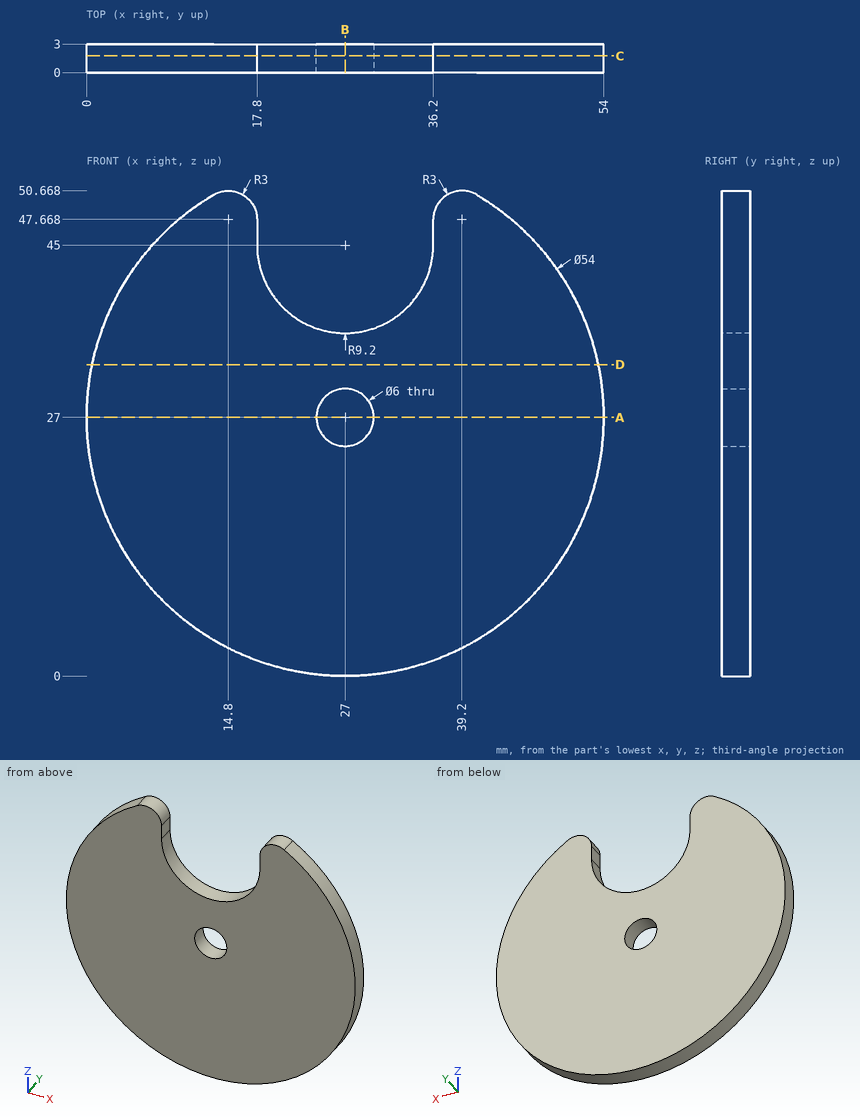
Job drawing, mm, ordinate dimensions from the low corner. One solid piece. Round coordinates to 2 decimals unless told otherwise and drop trailing zeros. Loops run counter-clockwise (first coordinate to the right, second up) from the corner with the lowest first, then second, coordinate; pieces in that order, holes last.
Item 1: Cut at A-A, the plane z = 27. Give the cut face in (x, y), then the cut area to 3 significant figures.
Item 2: Cut at D-D, the plane z = 32.5. Give the cut face in (x, y).
Item 3: Cut at B-B, the plane x = 27. Give the cut face in (y, z), then the cut area to 3 significant figures.
Item 4: Cut at C-C, the plane y = 1.75. Give the cut face in (x, z) (1 decimal), then the cut area to 3 significant figures.
Item 5: Drop a flat-ended pin along its axis: P1, Ø1.3, axis at y = 2, z = 46.5, coming from the -X side. Give the stop position or say it passes through.
Item 6: Drill centre lines: line 1 (Z direction, x = 27, y = 0.95); line 2 (Z direction, x = 29, y = 1.3) (1 decimal); line 3 (X direction, y = 0.55, z = 41.5). Where is each one in solid material? Low to high.
A:
1. outline: (0, 0) - (24, 0) - (24, 3) - (0, 3) - close; (30, 0) - (54, 0) - (54, 3) - (30, 3) - close
1. area: 144 mm2
2. outline: (0.57, 0) - (53.43, 0) - (53.43, 3) - (0.57, 3) - close
3. outline: (0, 0) - (3, 0) - (3, 24) - (0, 24) - close; (0, 30) - (3, 30) - (3, 35.8) - (0, 35.8) - close
3. area: 89.4 mm2
4. outline: (13.3, 50.3) arc R27 ccw (long way) to (40.7, 50.3) arc R3 ccw to (36.2, 47.7) - (36.2, 45) arc R9.2 cw to (17.8, 45) - (17.8, 47.7) arc R3 ccw to start; hole circle Ø6 at (27, 27)
4. area: 1,960 mm2
5. P1: stops at x = 7.67
6. line 1: z = 0 to 24, 30 to 35.8
6. line 2: z = 0.1 to 24.8, 29.2 to 36
6. line 3: x = 4.22 to 18.49, 35.51 to 49.78
